Could you check a few things on this model? Use its own coordinates, in mm. Face numbers are marked on the shaded views. A direction names the side the tool comes from. Give positions to 0.01 mm unless a question says otherwise; leave off trailing zeros. Loops run counter-clockwise (first coordinate to the right, second up) from the corner with the lowest first, then second, coordinate; pieces in that order, holes last. Notation, with made-up numbers: M 34.5,-28.75 L 52.5,-28.75 A14 ccw 52.5,-10.75 Z; hole C 6.25,60.5 d4. An arc over 180 degrees is marked long. Use a Markdown table: item, result. Add a question column.
1) If I drill on line 1 along Z through (x, y) = (-23, 1.65); line 2 along Z through (x, y) = (2, 1.75); line 3 along X through (y, z) = (1.55, -5.5), over which ranges is the centre line in solid material (lowest first)? Write a range as [from, to].
2) Will these pins go through, and if not, where does the flat tip stop? pin 1 Ø6 at (x, y) = (2, 2) entering from +Z; pin 2 Ø3.5 at (x, z) = (-2, 1) entering from -Y; pin 3 Ø5 at (x, z) = (-26.5, -1) entering from -Y; pin 4 Ø1.8 at (x, z) = (-32.5, 0) entering from -Y.
3) Suppose I cut it at D-D on x = -20. List the corners of the cut face in (y, z) for me, and give its area (3 significant figures).
4) Which directions (+Z, -Z, +X, -X, +Y, -Y) give clear straight access to the entire face, cutting with the end or side of a thin tool? Please do the marked faces 4, 5 and 6.
5) Suppose I cut it at C-C on z = 0. Count the separate pieces of the cut face and the enclosed holes in it, and give its area (3 significant figures).
6) Suppose I cut it at A-A on x = 15. List the corners of the cut face in (y, z) for me, and give its area (3 significant figures).
7) We'd pull the mould along X, two halves only. Please class the marked faces 1, 2 and 3: +X half, -X half, draft (parallel to the pull), parting line (faces both ways), or undercut.
8) Suppose I cut it at B-B on y = 3.5. List the corners of the cut face in (x, z) for me.
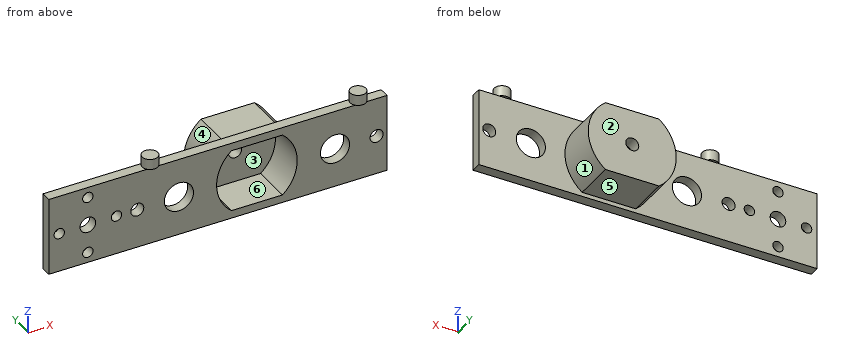
```python
from build123d import *

# Parameters (mm, degrees)
SKETCH_1_W               = 65
SKETCH_1_H               = 15
EXTRUDE_1_DEPTH          = 2
SKETCH_2_R               = 1.25
SKETCH_2_R_2             = 2.8
SKETCH_2_R_3             = 1.5
SKETCH_2_R_4             = 1
CUT_EXTRUDE_1_DEPTH      = 2
SKETCH_4_R               = 1.5
EXTRUDE_2_DEPTH          = 2
EXTRUDE_3_DEPTH          = 8
SKETCH_5_8_R             = 1.25
EXTRUDE_4_DEPTH          = 8
CUT_EXTRUDE_2_DEPTH      = 5.5
CUT_EXTRUDE_2_DEPTH_BACK = 42.883767739
SKETCH_5_11_R            = 1.25


with BuildPart() as part:
    # 草图1 → 凸台-拉伸1 (new body)
    with BuildSketch(Plane(origin=(0, 0, 0), x_dir=(1, 0, 0), z_dir=(0, 1, 0))):
        with Locations((-7.5, 0)):
            Rectangle(SKETCH_1_W, SKETCH_1_H)
    extrude(amount=EXTRUDE_1_DEPTH)

    # 草图2 → 切除-拉伸1 (cut)
    with BuildSketch(Plane(origin=(0, 0, 0), x_dir=(1, 0, 0), z_dir=(0, 1, 0))):
        with Locations(Location((0, 0, 0), (0, 0, 270))):
            Circle(SKETCH_2_R)
        with Locations(Location((15, 0, 0), (0, 0, 270))):
            Circle(SKETCH_2_R_2)
        with Locations(Location((-15, 0, 0), (0, 0, 90))):
            Circle(SKETCH_2_R_2)
        with Locations(Location((23, 0, 0), (0, 0, 270))):
            Circle(SKETCH_2_R)
        with Locations(Location((-23, 0, 0), (0, 0, 90))):
            Circle(SKETCH_2_R)
        with Locations(Location((-32.5, 0, 0), (0, 0, 270))):
            Circle(SKETCH_2_R_3)
        with Locations(Location((-27, 0, 0), (0, 0, 270))):
            Circle(SKETCH_2_R_4)
        with Locations(Location((-32.5, -5.5, 0), (0, 0, 270))):
            Circle(SKETCH_2_R_4)
        with Locations(Location((-38, 0, 0), (0, 0, 270))):
            Circle(SKETCH_2_R_4)
        with Locations(Location((-32.5, 5.5, 0), (0, 0, 270))):
            Circle(SKETCH_2_R_4)
    extrude(amount=CUT_EXTRUDE_1_DEPTH, mode=Mode.SUBTRACT)

    # 草图4 → 凸台-拉伸2 (add)
    with BuildSketch(Plane.XY.offset(7.5)):
        with Locations(Location((20, 1, 0), (0, 0, 221.810314896))):
            Circle(SKETCH_4_R)
        with Locations(Location((-20, 1, 0), (0, 0, 221.810314896))):
            Circle(SKETCH_4_R)
    extrude(amount=EXTRUDE_2_DEPTH)

    # 草图5 → 凸台-拉伸3 (add)
    with BuildSketch(Plane(origin=(0, 2, 0), x_dir=(1, 0, 0), z_dir=(0, 1, 0))):
        with BuildLine():
            Line((5.149029035, -6.7), (-5.149029035, -6.7))
            ThreePointArc((-5.149029035, -6.7), (-8.45, 0), (-5.149029035, 6.7))
            Line((-5.149029035, 6.7), (5.149029035, 6.7))
            ThreePointArc((5.149029035, 6.7), (8.45, 0), (5.149029035, -6.7))
        make_face()
        with BuildLine():
            Line((4.905354218, -6), (-4.905354218, -6))
            ThreePointArc((-4.905354218, -6), (-7.75, 0), (-4.905354218, 6))
            Line((-4.905354218, 6), (4.905354218, 6))
            ThreePointArc((4.905354218, 6), (7.75, 0), (4.905354218, -6))
        make_face(mode=Mode.SUBTRACT)
    extrude(amount=EXTRUDE_3_DEPTH)

    # 草图5<8> → 凸台-拉伸4 (add)
    with BuildSketch(Plane(origin=(0, 2, 0), x_dir=(1, 0, 0), z_dir=(0, 1, 0))):
        with BuildLine():
            Line((4.905354218, -6), (-4.905354218, -6))
            ThreePointArc((-4.905354218, -6), (-7.75, 0), (-4.905354218, 6))
            Line((-4.905354218, 6), (4.905354218, 6))
            ThreePointArc((4.905354218, 6), (7.75, 0), (4.905354218, -6))
        make_face()
        with Locations(Location((0, 0, 0), (0, 0, 270))):
            Circle(SKETCH_5_8_R, mode=Mode.SUBTRACT)
    extrude(amount=EXTRUDE_4_DEPTH)

    # 草图5<11> → 切除-拉伸2 (cut, two sides: drawn at the far end of the back side and taken through both)
    with BuildSketch(Plane(origin=(0, 2, 0), x_dir=(1, 0, 0), z_dir=(0, 1, 0)).offset(-CUT_EXTRUDE_2_DEPTH_BACK)):
        with BuildLine():
            Line((4.905354218, -6), (-4.905354218, -6))
            ThreePointArc((-4.905354218, -6), (-7.75, 0), (-4.905354218, 6))
            Line((-4.905354218, 6), (4.905354218, 6))
            ThreePointArc((4.905354218, 6), (7.75, 0), (4.905354218, -6))
        make_face()
        with Locations(Location((0, 0, 0), (0, 0, 270))):
            Circle(SKETCH_5_11_R, mode=Mode.SUBTRACT)
    extrude(amount=CUT_EXTRUDE_2_DEPTH + CUT_EXTRUDE_2_DEPTH_BACK, mode=Mode.SUBTRACT)


solid = part.part
```
Answer block:
| question | item | result |
|---|---|---|
| 1 | line 1 | z = [-7.5, -1.25], [1.25, 7.5] |
| 1 | line 2 | z = [-7.5, -6], [6, 7.5] |
| 1 | line 3 | x = [-40, -33.5], [-31.5, -5.46], [5.46, 25] |
| 2 | pin 1 | stops at z = 7.5 |
| 2 | pin 2 | stops at y = 7.5 |
| 2 | pin 3 | stops at y = 0 |
| 2 | pin 4 | passes through |
| 3 | outline | M -0.5,7.5 L 0,7.5 L 0,-7.5 L 2,-7.5 L 2,7.5 L 2.5,7.5 L 2.5,9.5 L -0.5,9.5 Z |
| 3 | area | 36.0 mm^2 |
| 4 | face 4 | -X, +Y |
| 4 | face 5 | -Z, +X, -X, +Y |
| 4 | face 6 | -Y |
| 5 | separate pieces | 9 |
| 5 | enclosed holes | 0 |
| 5 | area | 96.3 mm^2 |
| 6 | outline | M 0,-7.5 L 2,-7.5 L 2,-2.8 L 0,-2.8 Z; M 0,2.8 L 2,2.8 L 2,7.5 L 0,7.5 Z |
| 6 | area | 18.8 mm^2 |
| 7 | face 1 | +X half |
| 7 | face 2 | draft |
| 7 | face 3 | undercut |
| 8 | outline | M -5.15,-6.7 L 5.15,-6.7 A8.45 ccw 5.15,6.7 L -5.15,6.7 A8.45 ccw Z; hole M -4.91,-6 L 4.91,-6 A7.75 ccw 4.91,6 L -4.91,6 A7.75 ccw Z |
